Can you work these out from the model? Positions are in its coordinate system, mm. A direction names the side the tool comes from. Coordinates: 2 decimals unless noted, no trailing zeros. Order: outer loops, then holes, each group sorted by start corner. A loop starts at its lowest first (then second) coordinate and runs counter-clockwise, first axis right, second up. Notation, with made-up numbers: (-24, 59.25) -> (12, 59.25) arc R17 cw to (12, 85.25) -> close; hole circle Ø2 at (-5, 10). An arc over 180 degrees is marked (long way). Write item = value, one per line.
```python
from build123d import *

# Parameters (mm, degrees)
EXTRUDE_1_DEPTH     = 260
SKETCH_4_R          = 1.5
CUT_EXTRUDE_3_DEPTH = 6
SKETCH_5_R          = 1.5
CUT_EXTRUDE_4_DEPTH = 4


with BuildPart() as part:
    # Эскиз1 → Бобышка-Вытянуть1 (new body)
    with BuildSketch(Plane(origin=(0, 0, 0), x_dir=(0, 0, -1), z_dir=(1, 0, 0))):
        Polygon((0, 0), (-11, 0), (-11, 3), (-5, 3), (-5, 9.5), (-2, 9.5), (-2, 11), (0, 11), align=None)
    extrude(amount=EXTRUDE_1_DEPTH)

    # Эскиз4 → Вырез-Вытянуть3 (cut, through all)
    with BuildSketch(Plane.XY.offset(5)):
        with Locations((42, 5.4)):
            Circle(SKETCH_4_R)
        with Locations((218, 5.4)):
            Circle(SKETCH_4_R)
    extrude(amount=-CUT_EXTRUDE_3_DEPTH, mode=Mode.SUBTRACT)

    # Эскиз5 → Вырез-Вытянуть4 (cut, through all)
    with BuildSketch(Plane(origin=(0, 3, 0), x_dir=(1, 0, 0), z_dir=(0, 1, 0))):
        with Locations((26.91, -6.8)):
            Circle(SKETCH_5_R)
        with Locations((233.09, -6.8)):
            Circle(SKETCH_5_R)
    extrude(amount=-CUT_EXTRUDE_4_DEPTH, mode=Mode.SUBTRACT)


solid = part.part
```
Item 1: I'm going to push flat-ended pins straight in: P1, Ø5, axis at x = 164.5, y = 8, coming from the +Z side; P2, Ø2.5, axis at x = 26.91, z = 6.8, coming from the -Y side; P3, Ø6.5, axis at x = 88.5, z = 8.5, coming from the +Y side. Where does each tip first touch, or does it pass through?
A:
P1 = 5
P2 = through
P3 = 3
Item 2: For faces 1 (the flat face through (128, 3, 8)), 2 (the flat face through (260, 4, 3)), which set-ups out of +Z, -Z, +X, -X, +Y, -Y let a thin tool reach every point of the face, with its end or its side?
A:
face_1 = +Z, +X, -X, +Y
face_2 = +Z, -Z, +X, +Y, -Y
Item 3: I want a section at A-A, the plane x = 106. Please give me the cut outline in (y, z).
A:
outline = (0, 0) -> (11, 0) -> (11, 2) -> (9.5, 2) -> (9.5, 5) -> (3, 5) -> (3, 11) -> (0, 11) -> close
Item 4: If I drill on probe 1 along X at (y, z) = (1, 6.8); probe 2 along Z at (x, y) = (233.09, 2.05); probe 3 along Y at (x, z) = (218, 2.55), over which ranges is the centre line in solid material (lowest first)?
A:
probe_1 = 0 to 25.41, 28.41 to 231.59, 234.59 to 260
probe_2 = 0 to 5.3, 8.3 to 11
probe_3 = 0 to 3.9, 6.9 to 9.5
